Work out the finished part from the listing and answer in its coordinate system (mm). A direction names the side the tool comes from. Coordinates: 2 decimals unless noted, no trailing zeros. Loops run counter-clockwise (first coordinate to the right, second up) from the corner with the lowest first, then second, coordinate; pieces in that order, holes last. Notation, with made-up numbers: (-30.75, 79) - (-21.75, 79) arc R21 ccw to (-21.75, 89) - close; hole circle Ø6 at (31, 8.5). An arc over 180 degrees is marked (long way). Write each question's results on one line, items separated by ' | '. Start each with the question number.
Item 1: Each of these flat-tipped pins is pushed along its axis until it touches: pin 1 Ø2 at (x, z) = (6, 60) entering from -Y; pin 2 Ø1 at (y, z) = (-4.5, 22.5) entering from +X; pin 3 Ø1.5 at (y, z) = (-2, 39) entering from +X. Where does it stop, or does it pass through?
Item 2: Section A-A, the plane y = -1.75 is taken. Write down the section's boundary in (x, z), plus the area to 3 significant figures.
Item 3: For a pull along X with two mould halves and no side action, classify faces 3 (the face through (5, 0, 35)), 4 (the face through (5, 0.9, 35)) as +X half, -X half, draft (parallel to the pull), parting line (faces both ways), or undercut.
Item 4: Section C-C, the plane z = 58 is taken. Write down the section's boundary in (x, y).
Item 5: A tool of negligible diameter and unlimited length cuts with its end or side. For faces 1 (the face through (0.996, -2.479, 34.51)), 2 (the face through (4.6, 0.3, 0)), from which of +Z, -Z, +X, -X, +Y, -Y can it reach the whole face along a straight path? Write none if from no direction.
Item 6: Consider probe 1 along X at (y, z) = (-2.25, 5); probe 2 along Y at (x, z) = (7.5, 58); probe 3 along X at (y, z) = (-1.75, 62.5). Determine where each line is inside the solid, lowest interval first. Write a range as [from, to].
Item 7: Section B-B, the plane x = 2.5 is taken. Write down the section's boundary in (y, z).
from build123d import *

# Parameters (mm, degrees)
EXTRUDE_1_DEPTH = 70


with BuildPart() as part:
    # 草图1 → 凸台-拉伸1 (new body)
    with BuildSketch(Plane.XY):
        with BuildLine():
            Line((0.2, 0.9), (9.6, 0.9))
            ThreePointArc((9.6, 0.9), (9.741421356, 0.841421356), (9.8, 0.7))
            Line((9.8, 0.7), (9.8, 0))
            Line((9.8, 0), (9.095909231, 0))
            ThreePointArc((9.095909231, 0), (9.703179683, -2.690137412), (8.967513749, -5.348033635))
            ThreePointArc((8.967513749, -5.348033635), (8.857560706, -5.459239359), (8.706580725, -5.5))
            Line((8.706580725, -5.5), (8.358309598, -5.5))
            ThreePointArc((8.358309598, -5.5), (8.096544276, -5.34655687), (8.10255289, -5.043192773))
            ThreePointArc((8.10255289, -5.043192773), (8.804655076, -2.515755891), (8.061784314, 0))
            Line((8.061784314, 0), (1.738215686, 0))
            ThreePointArc((1.738215686, 0), (0.995344924, -2.515755891), (1.69744711, -5.043192773))
            ThreePointArc((1.69744711, -5.043192773), (1.703455724, -5.34655687), (1.441690402, -5.5))
            Line((1.441690402, -5.5), (1.093419275, -5.5))
            ThreePointArc((1.093419275, -5.5), (0.942439294, -5.459239359), (0.832486251, -5.348033635))
            ThreePointArc((0.832486251, -5.348033635), (0.096820317, -2.690137412), (0.704090769, 0))
            Line((0.704090769, 0), (0, 0))
            Line((0, 0), (0, 0.7))
            ThreePointArc((0, 0.7), (0.058578644, 0.841421356), (0.2, 0.9))
        make_face()
    extrude(amount=EXTRUDE_1_DEPTH)


solid = part.part
Answer key:
1) pin 1: stops at y = 0 | pin 2: stops at x = 9.52 | pin 3: stops at x = 9.7
2) outline: (0.15, 0) - (1.06, 0) - (1.06, 70) - (0.15, 70) - close; (8.74, 0) - (9.65, 0) - (9.65, 70) - (8.74, 70) - close | area: 128 mm^2
3) face 3: undercut | face 4: draft
4) outline: (0, 0) - (0.7, 0) arc R5.66 ccw to (0.83, -5.35) arc R0.3 ccw to (1.09, -5.5) - (1.44, -5.5) arc R0.3 ccw to (1.7, -5.04) arc R4.76 cw to (1.74, 0) - (8.06, 0) arc R4.76 cw to (8.1, -5.04) arc R0.3 ccw to (8.36, -5.5) - (8.71, -5.5) arc R0.3 ccw to (8.97, -5.35) arc R5.66 ccw to (9.1, 0) - (9.8, 0) - (9.8, 0.7) arc R0.2 ccw to (9.6, 0.9) - (0.2, 0.9) arc R0.2 ccw to (0, 0.7) - close
5) face 1: +Z, -Z | face 2: -Z, +X, -X, +Y, -Y
6) probe 1: x = [0.1, 1], [8.8, 9.7] | probe 2: y = [0, 0.9] | probe 3: x = [0.15, 1.06], [8.74, 9.65]
7) outline: (0, 0) - (0.9, 0) - (0.9, 70) - (0, 70) - close
